from build123d import *

# Parameters (mm, degrees)
SKETCH018_R     = 4.25
SKETCH018_R_2   = 9
SKETCH018_W     = 6
SKETCH018_H     = 3
PAD011_DEPTH    = 8
SKETCH020_W     = 56.576859
SKETCH020_H     = 40
POCKET007_DEPTH = 4.5
POCKET008_DEPTH = 4.5
SKETCH021_R     = 9
PAD012_DEPTH    = 3.5
POCKET009_DEPTH = 20.001


with BuildPart() as part:
    # Sketch018 → Pad011 (new body)
    with BuildSketch(Plane.XY):
        with BuildLine():
            Line((20, 58), (20, -13))
            ThreePointArc((13, -20), (17.949747, -17.949747), (20, -13))
            Line((13, -20), (-73, -20))
            ThreePointArc((-80, -13), (-77.949747, -17.949747), (-73, -20))
            Line((-80, -13), (-80, 71))
            ThreePointArc((-73, 78), (-77.949747, 75.949747), (-80, 71))
            Line((-73, 78), (-22, 78))
            Line((-22, 31), (-22, 78))
            Line((-73, 31), (-22, 31))
            ThreePointArc((-73, 31), (-74.767767, 30.267767), (-75.5, 28.5))
            Line((-75.5, 28.5), (-75.5, -13))
            ThreePointArc((-75.5, -13), (-73.751764, -15.384292), (-70.95212, -14.433941))
            Line((-70.95212, -14.433941), (-43.329649, 25.015035))
            ThreePointArc((-37.595585, 28), (-40.827825, 27.209076), (-43.329649, 25.015035))
            Line((-37.595585, 28), (-22, 28))
            ThreePointArc((-22, 28), (-17.050253, 30.050253), (-15, 35))
            Line((-15, 35), (-15, 58))
            ThreePointArc((-8, 65), (-12.949747, 62.949747), (-15, 58))
            Line((-8, 65), (13, 65))
            ThreePointArc((20, 58), (17.949747, 62.949747), (13, 65))
        make_face()
        Circle(SKETCH018_R, mode=Mode.SUBTRACT)
        with Locations((4, 46)):
            Circle(SKETCH018_R_2, mode=Mode.SUBTRACT)
        with BuildLine():
            ThreePointArc((-38, 63), (-47, 54), (-38, 45))
            Line((-38, 45), (-35, 45))
            ThreePointArc((-35, 45), (-26, 54), (-35, 63))
            Line((-35, 63), (-38, 63))
        make_face(mode=Mode.SUBTRACT)
        with BuildLine():
            ThreePointArc((-67, 70), (-69, 68), (-67, 66))
            Line((-67, 66), (-64, 66))
            ThreePointArc((-64, 66), (-62, 68), (-64, 70))
            Line((-64, 70), (-67, 70))
        make_face(mode=Mode.SUBTRACT)
        with BuildLine():
            ThreePointArc((-67, 42), (-69, 40), (-67, 38))
            Line((-67, 38), (-64, 38))
            ThreePointArc((-64, 38), (-62, 40), (-64, 42))
            Line((-64, 42), (-67, 42))
        make_face(mode=Mode.SUBTRACT)
        with Locations((6, 34.5)):
            Rectangle(SKETCH018_W, SKETCH018_H, mode=Mode.SUBTRACT)
        with Locations((-6, 34.5)):
            Rectangle(SKETCH018_W, SKETCH018_H, mode=Mode.SUBTRACT)
    extrude(amount=PAD011_DEPTH)

    # Sketch020 → Pocket007 (cut)
    with BuildSketch(Plane.XY):
        with Locations((-47.711571, 54)):
            Rectangle(SKETCH020_W, SKETCH020_H)
    extrude(amount=POCKET007_DEPTH, mode=Mode.SUBTRACT)

    # Sketch019 (on Face5 of Pocket007) → Pocket008 (cut)
    with BuildSketch(Plane.XY.offset(8)):
        Polygon((-73, -15.5), (-25.471525, -15.5), (-25.471525, -22.26432), (22.647079, -22.26432), (22.647079, 72.273804), (-17.92174, 72.273804), (-17.92174, 30.299976), (-42.694947, 30.299976), (-73, -13), align=None)
    extrude(amount=-POCKET008_DEPTH, mode=Mode.SUBTRACT)

    # Sketch021 (on Face38 of Pocket008) → Pad012 (join)
    with BuildSketch(Plane.XY.offset(8)):
        with BuildLine():
            ThreePointArc((-7.496085, 26.109881), (24.755897, 32.411198), (14.768623, 63.718565))
            Line((-13.056022, 76.099882), (14.768623, 63.718565))
            ThreePointArc((-13.056022, 76.099882), (-17.428206, 77.519728), (-22, 78))
            Line((-22, 78), (-22, 31))
            ThreePointArc((-7.496085, 26.109881), (-14.346948, 29.744572), (-22, 31))
        make_face()
        with Locations((5.824645, 43.618683)):
            Circle(SKETCH021_R, mode=Mode.SUBTRACT)
    extrude(amount=-PAD012_DEPTH)

    # Sketch022 → Pocket009 (cut, through all)
    with BuildSketch(Plane.XZ):
        Polygon((0, 3), (-25, 3), (-40.931572, 8.439757), (-40.931572, 13.093841), (-0.040726, 13.093841), align=None)
    extrude(amount=POCKET009_DEPTH, mode=Mode.SUBTRACT)


with BuildPart() as part_1:
    # Body008 placement: moved
    add(part.part.moved(Location((0, 0, 0.5))))


solid = part_1.part
Input: part model. Units: mm. Frame: model coordinates. A direction names the side the tool comes from. Give positions to 0.01 mm unless a question says otherwise; leave off trailing zeros. Write each loop counter-clockwise with the first axis right and the second up, starting at its lowest first coordinate (ties: lowest second). Pieces come first, ordered by that corner, then holes. Notation, with made-up numbers: (36.25, 42.5) -> (53.25, 42.5) arc R19 ccw to (53.25, 48.5) -> close; hole circle Ø5 at (-8.75, 60.5). An arc over 180 degrees is marked (long way). Use one line per item in the form item = value. Start each with the question number.
1) Ray query, probe 1 along X at (y, z) = (46, 1.85); probe 2 along X at (y, z) = (52, 3.5); probe 3 along Z at (x, y) = (-16.5, -7.5). Return the intervals inside material, ascending. Write a range as from..to.
2) Draft query along X for faces 4 (the cylindrical face through (18, 62.9, 2.2)), 5 (the cylindrical face through (3.874, 34.833, 6.774)), 6 (the flat face through (-30, 28, 2)), 7 (the cylindrical face through (-77.9, 76, 4.4)). Return one class per face: pulls with the +X half, pulls with the -X half, needs draft (parallel to the pull), parting line crosses it, or undercut.
3) Section query D-D on y = 68. Return the cut outline in (x, z), then the cut area to 3 significant figures.
4) Section query A-A on y = -8.5. Return the cut outline in (x, z).
5) Section query B-B on z = 2.25. Count the separate pieces of the cut face and the enclosed holes in it, then the cut area to 3 significant figures.
6) Set-up query: faces 1 (the cylindrical face through (2.828, 54.923, 2.226)), 2 (the cylindrical face through (-47, 54, 7)), 3 (the flat face through (-12, -10, 3.5)). Return all of +Z, -Z, +X, -X, +Y, -Y with unobstructed straight access to the full face (end or side cutting, diameter ignored); none if empty.
7) Pin query (flat end, axial travel): pin 1 (1.8 mm diameter, centred on x = 5, z = 2.5, fed in from +Y); pin 2 (1.5 mm diameter, centred on y = 56, z = 2.5, fed in from +X); pin 3 (1 mm diameter, centred on x = 13, z = 6, fed in from +Y). Return the tip coordinate at first contact, or that it passes through.
8) Section query C-C on y = 40. Return the cut outline in (x, z) (3 decimals), then the cut area to 3 significant figures.
Outcome:
q1.probe_1 = -80..-76, -15..-5, 13..20
q1.probe_2 = -80..-76, -15..-2.71, 10.71..20
q1.probe_3 = 0.5..3.5
q2.face_4 = pulls with the +X half
q2.face_5 = undercut
q2.face_6 = undercut
q2.face_7 = pulls with the -X half
q3.outline = (-80, 0.5) -> (-76, 0.5) -> (-76, 5) -> (-69, 5) -> (-69, 8.5) -> (-80, 8.5) -> close; (-62, 5) -> (5.15, 5) -> (5.15, 8.5) -> (-62, 8.5) -> close
q3.area = 292 mm^2
q4.outline = (-80, 0.5) -> (-75.5, 0.5) -> (-75.5, 8.5) -> (-80, 8.5) -> close; (-66.8, 0.5) -> (20, 0.5) -> (20, 4) -> (0, 4) -> (0, 3.5) -> (-25, 3.5) -> (-26.46, 4) -> (-66.8, 4) -> close
q5.separate_pieces = 1
q5.enclosed_holes = 4
q5.area = 5,460 mm^2
q6.face_1 = -Z
q6.face_2 = +Z, -Z
q6.face_3 = +Z, -Y
q7.pin_1 = 65
q7.pin_2 = 20
q7.pin_3 = 64.73
q8.outline = (-80, 0.5) -> (-76, 0.5) -> (-76, 5) -> (-69, 5) -> (-69, 8.5) -> (-80, 8.5) -> close; (-62, 5) -> (-2.416, 5) -> (-2.416, 8.5) -> (-62, 8.5) -> close; (-15, 0.5) -> (-2.708, 0.5) -> (-2.708, 4) -> (-15, 4) -> close; (10.708, 0.5) -> (20, 0.5) -> (20, 4) -> (10.708, 4) -> close; (14.065, 5) -> (27.525, 5) -> (27.525, 8.5) -> (14.065, 8.5) -> close
q8.area = 388 mm^2
